```python
from build123d import *

# Parameters (mm, degrees)
SKETCH1_W           = 50.8
SKETCH1_H           = 5
BOSS_EXTRUDE1_DEPTH = 10
CUT_EXTRUDE2_DEPTH  = 53.01576684
LPATTERN1_COUNT     = 4
LPATTERN1_PITCH     = 12.7


with BuildPart() as part:
    # Sketch1 → Boss-Extrude1 (new body)
    with BuildSketch(Plane.XY):
        with Locations((25.4, 2.5)):
            Rectangle(SKETCH1_W, SKETCH1_H)
    extrude(amount=BOSS_EXTRUDE1_DEPTH)

    # Sketch3 → Cut-Extrude2 (cut, through all)
    with BuildSketch(Plane.XY.offset(10)):
        Polygon((2.008089297, 8), (4.191910703, 2), (8.508089297, 2), (10.691910703, 8), align=None)
    cut_extrude2 = extrude(amount=-CUT_EXTRUDE2_DEPTH, mode=Mode.SUBTRACT)

    # LPattern1: Cut-Extrude2 ×4
    with Locations(*[(i * LPATTERN1_PITCH, 0, 0) for i in range(1, LPATTERN1_COUNT)]):
        add(cut_extrude2, mode=Mode.SUBTRACT)


solid = part.part
```
Verification items for the finished model (mm, model axes). A direction names the side the tool comes from. Coordinates: 2 decimals unless noted, no trailing zeros. Order: outer loops, then holes, each group sorted by start corner. A loop starts at its lowest first (then second) coordinate and runs counter-clockwise, first axis right, second up. Notation, with made-up numbers: (74, 63.25) - (99, 63.25) arc R16 cw to (99, 71.25) - close; hole circle Ø1 at (20.25, -25.75). An arc over 180 degrees is marked (long way). Return JSON: item names as keys, results as strings.
(1) Thickness scan on line 1 along X through (y, z) = (3.9, 1.5); line 2 along X through (y, z) = (2.5, 2.25); line 3 along Y through (x, z) = (21, 7.5). Record the ranges inside material, lowest first.
Filled sheet:
{"line 1": "x = 0 to 3.5, 9.2 to 16.2, 21.9 to 28.9, 34.6 to 41.6, 47.3 to 50.8", "line 2": "x = 0 to 4.01, 8.69 to 16.71, 21.39 to 29.41, 34.09 to 42.11, 46.79 to 50.8", "line 3": "y = 0 to 2"}
(2) Section check B-B, the plane x = 33. Record the cut outline in (y, z), and give its area (3 significant figures).
Filled sheet:
{"outline": "(0, 0) - (2, 0) - (2, 10) - (0, 10) - close", "area": "20.0 mm^2"}
(3) Mould release check, pull along X, two halves, no side actions. Record for faces 3 (the flat face through (50.8, 2, 5)), 4 (the flat face through (38, 5, 5)), 5 (the flat face through (29.04, 3.52, 5.07)): pulls with the +X half, pulls with the -X half, needs draft (parallel to the pull), parting line crosses it, or undercut.
Filled sheet:
{"face 3": "pulls with the +X half", "face 4": "needs draft", "face 5": "undercut"}
(4) Access from +Z, -Z, +X, -X, +Y, -Y to the whole of each face (thin tool, end or side, straight path). Record for faces 1 (the flat face through (25, 2, 10)), 2 (the flat face through (47.146, 3.479, 5.07)).
Filled sheet:
{"face 1": "+Z, +X, -X, +Y, -Y", "face 2": "+Z, -Z, +Y"}
(5) Section check A-A, the plane y = 3.1. Record the cut outline in (x, z), and give its area (3 significant figures).
Filled sheet:
{"outline": "(0, 0) - (3.79, 0) - (3.79, 10) - (0, 10) - close; (8.91, 0) - (16.49, 0) - (16.49, 10) - (8.91, 10) - close; (21.61, 0) - (29.19, 0) - (29.19, 10) - (21.61, 10) - close; (34.31, 0) - (41.89, 0) - (41.89, 10) - (34.31, 10) - close; (47.01, 0) - (50.8, 0) - (50.8, 10) - (47.01, 10) - close", "area": "303 mm^2"}
(6) Go/stop test with a flat-tipped pin: pin 1 (2 mm diameter, centred on x = 6, z = 5.5, fed in from +Y). Record where the tip stops, or that it passes through.
Filled sheet:
{"pin 1": "stops at y = 2"}
